Part print with two shaded views. Sizes in mm from the minimum x, y, z corner. A direction names the side the tool comes from. Coordinates: 2 decimals unless noted, no trailing zeros. Loops run counter-clockwise (first coordinate to the right, second up) from the corner with the lowest first, then second, coordinate; pieces in that order, holes last. Notation, with made-up numbers: (-26.75, 7.5) -> (11.25, 7.5) arc R33 ccw to (11.25, 35.5) -> close; hole circle Ø6 at (83, 79.5). An arc over 180 degrees is marked (long way). Use one line per item in the form item = value.
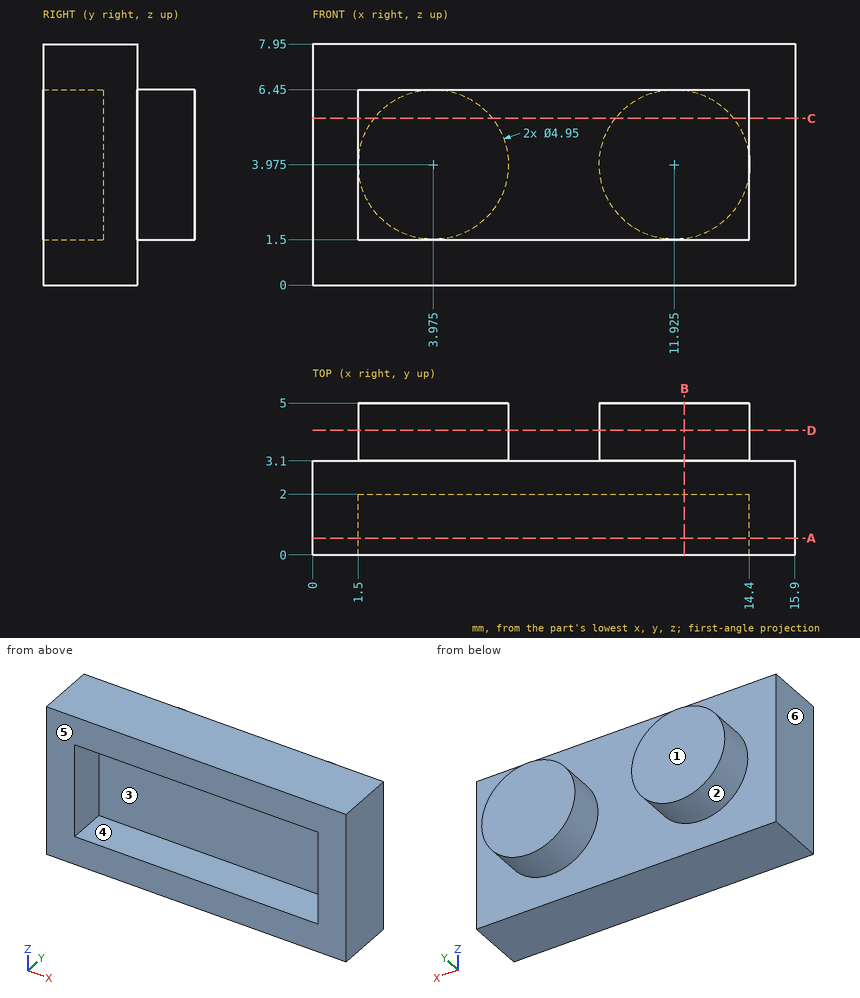
Q1. Band-saw the part on A-A, the plane y = 0.55. Write the cut outline in (x, z), and give its area (4 significant figures).
Result:
outline = (0, 0) -> (15.9, 0) -> (15.9, 7.95) -> (0, 7.95) -> close; hole (1.5, 1.5) -> (14.4, 1.5) -> (14.4, 6.45) -> (1.5, 6.45) -> close
area = 62.55 mm2
Q2. Mould opens along X. For the marked faces 4, 5 and 6 say: released by +X, released by -X, zero draft, split by the parting line, or undercut.
Result:
face_4 = undercut
face_5 = zero draft
face_6 = released by -X
Q3. Band-saw the part on C-C, the plane z = 5.5. Write the cut outline in (x, y), and give its area (3 significant figures).
Result:
outline = (0, 0) -> (1.5, 0) -> (1.5, 2) -> (14.4, 2) -> (14.4, 0) -> (15.9, 0) -> (15.9, 3.1) -> (13.87, 3.1) -> (13.87, 5) -> (9.98, 5) -> (9.98, 3.1) -> (5.92, 3.1) -> (5.92, 5) -> (2.03, 5) -> (2.03, 3.1) -> (0, 3.1) -> close
area = 38.3 mm2
Q4. Pin check, flat tips, straight feed: pin 1 Ø2.5 at (x, z) = (5.5, 5) entering from -Y; pin 2 Ø1 at (y, z) = (1, 4.5) entering from -X. Stop position of each tip, or through.
Result:
pin_1 = 2
pin_2 = 0
Q5. Band-saw the part on D-D, the plane y = 4.1. Write the cut outline in (x, z) (3 decimals).
Result:
outline = circle Ø4.95 at (3.975, 3.975); circle Ø4.95 at (11.925, 3.975)
Q6. Band-saw the part on B-B, the plane x = 12.25. Write the cut outline in (y, z), and give its area (3 significant figures).
Result:
outline = (0, 0) -> (3.1, 0) -> (3.1, 1.52) -> (5, 1.52) -> (5, 6.43) -> (3.1, 6.43) -> (3.1, 7.95) -> (0, 7.95) -> (0, 6.45) -> (2, 6.45) -> (2, 1.5) -> (0, 1.5) -> close
area = 24.1 mm2
Q7. Which spindle directions (+Z, -Z, +X, -X, +Y, -Y) get a long thin tool onto all of the face, cutting with end or side? Do the marked faces 1, 2 and 3. Say none if no direction does.
Result:
face_1 = +Z, -Z, +X, -X, +Y
face_2 = +Y
face_3 = -Y
Q8. Wall check: line 1 along X through (y, z) = (0.4, 4.75); line 2 along Z through (x, y) = (4.5, 1.6); line 3 along Z through (x, y) = (4, 4.65). Give the ranges that are in metal, low to high.
Result:
line_1 = 0 to 1.5, 14.4 to 15.9
line_2 = 0 to 1.5, 6.45 to 7.95
line_3 = 1.5 to 6.45
